The listing builds one solid part. Answer for the finished solid, in the listing's coordinates (mm). Coordinates: 2 decimals unless noted, no trailing zeros. Loops run counter-clockwise (first coordinate to the right, second up) from the corner with the lowest first, then second, coordinate; pieces in that order, holes last. Notation, with made-up numbers: M 3,36.5 L 9,36.5 A17 ccw 9,51.5 Z; hole C 4.5,-18.5 d7. An arc over 180 degrees is marked long. Answer as a JSON object with one key per item and string values. Group by question number.
1. A cutting plane is placed at C-C on x = -40.5. Give the vertices of the cut face in (y, z).
2. Straight lines are drawn through the part: L1, parallel to Z at x = -2, y = 1.25; L2, parallel to Y at x = 7, z = -9; L3, parallel to Z at x = -8, y = 8.75. For each, find the intervals that lie inside material, in ascending order.
3. A cutting plane is placed at A-A on z = 0. Give the vertices of the cut face in (x, y).
4. A cutting plane is placed at B-B on y = 10. Give the vertices of the cut face in (x, z), and give its area (3 significant figures).
5. Given pin 1 (5 mm diameter, centred on x = 24, y = 1.5, fed in from -Z); pin 2 (6 mm diameter, centred on x = -27.5, y = 11, fed in from -Z); pin 3 (6 mm diameter, centred on x = 54.5, y = 7, fed in from -Z), each flat-ended and moving along its own axis, determine where each tip first touches the part or whether it passes through.
6. A cutting plane is placed at D-D on x = 33. Give the vertices of the cut face in (y, z), and give its area (3 significant figures).
from build123d import *

# Parameters (mm, degrees)
SKETCH1_R           = 70
BOSS_EXTRUDE1_DEPTH = 13
SKETCH2_R           = 10
CUT_EXTRUDE1_DEPTH  = 100.844879688
SKETCH3_R           = 8.334076576
CUT_EXTRUDE2_DEPTH  = 10.220805
CIRPATTERN1_START   = 2.779195168
CIRPATTERN1_DEPTH   = 10.220804832


# Read off the part's stored shape, not the designer's step: CirPattern1
with BuildPart() as part:
    # Sketch1 → Boss-Extrude1 (new body)
    with BuildSketch(Plane(origin=(0, 0, 0), x_dir=(1, 0, 0), z_dir=(0, 1, 0))):
        with Locations(Location((0, 0, 0), (0, 0, 90))):
            Circle(SKETCH1_R)
    extrude(amount=BOSS_EXTRUDE1_DEPTH)

    # Sketch2 → Cut-Extrude1 (cut, through all)
    with BuildSketch(Plane(origin=(0, 0, 0), x_dir=(1, 0, 0), z_dir=(0, 1, 0))):
        with Locations(Location((0, 0, 0), (0, 0, 90))):
            Circle(SKETCH2_R)
    extrude(amount=CUT_EXTRUDE1_DEPTH, mode=Mode.SUBTRACT)

    # Sketch3 → Cut-Extrude2 (cut)
    with BuildSketch(Plane(origin=(0, 13, 0), x_dir=(1, 0, 0), z_dir=(0, 1, 0))):
        with Locations((-16.463436294, 0)):
            Circle(SKETCH3_R)
    extrude(amount=-CUT_EXTRUDE2_DEPTH, mode=Mode.SUBTRACT)

    # CirPattern1 outline → CirPattern1 (cut)
    with BuildSketch(Plane(origin=(0, 0, 0), x_dir=(1, 0, 0), z_dir=(0, 1, 0)).offset(CIRPATTERN1_START)):
        with BuildLine():
            ThreePointArc((8.05530373, -5.925544854), (5, -8.660254038), (1.104020509, -9.938870092))
            ThreePointArc((1.104020509, -9.938870092), (0.405285183, -11.39353001), (0, -12.955583291))
            ThreePointArc((0, -12.955583291), (-0.405285183, -11.39353001), (-1.104020509, -9.938870092))
            ThreePointArc((-1.104020509, -9.938870092), (-5, -8.660254038), (-8.05530373, -5.925544854))
            ThreePointArc((-8.05530373, -5.925544854), (-9.664443836, -6.047752269), (-11.219864251, -6.477791645))
            ThreePointArc((-11.219864251, -6.477791645), (-12.296398006, -7.217522031), (-13.475290189, -7.779962418))
            ThreePointArc((-13.475290189, -7.779962418), (-12.398756435, -21.475276095), (0, -15.559924837))
            ThreePointArc((0, -15.559924837), (12.398756435, -21.475276095), (13.475290189, -7.779962418))
            ThreePointArc((13.475290189, -7.779962418), (24.797512869, 0), (13.475290189, 7.779962418))
            ThreePointArc((13.475290189, 7.779962418), (12.398756435, 21.475276095), (0, 15.559924837))
            ThreePointArc((0, 15.559924837), (-12.398756435, 21.475276095), (-13.475290189, 7.779962418))
            ThreePointArc((-13.475290189, 7.779962418), (-12.296398006, 7.217522031), (-11.219864251, 6.477791645))
            ThreePointArc((-11.219864251, 6.477791645), (-9.664443836, 6.047752269), (-8.05530373, 5.925544854))
            ThreePointArc((-8.05530373, 5.925544854), (-5, 8.660254038), (-1.104020509, 9.938870092))
            ThreePointArc((-1.104020509, 9.938870092), (-0.405285183, 11.39353001), (0, 12.955583291))
            ThreePointArc((0, 12.955583291), (0.405285183, 11.39353001), (1.104020509, 9.938870092))
            ThreePointArc((1.104020509, 9.938870092), (5, 8.660254038), (8.05530373, 5.925544854))
            ThreePointArc((8.05530373, 5.925544854), (9.664443836, 6.047752269), (11.219864251, 6.477791645))
            ThreePointArc((11.219864251, 6.477791645), (10.069729019, 5.345777741), (9.15932424, 4.013325239))
            ThreePointArc((9.15932424, 4.013325239), (10, 0), (9.15932424, -4.013325239))
            ThreePointArc((9.15932424, -4.013325239), (10.069729019, -5.345777741), (11.219864251, -6.477791645))
            ThreePointArc((11.219864251, -6.477791645), (9.664443836, -6.047752269), (8.05530373, -5.925544854))
        make_face()
    extrude(amount=CIRPATTERN1_DEPTH, mode=Mode.SUBTRACT)


solid = part.part
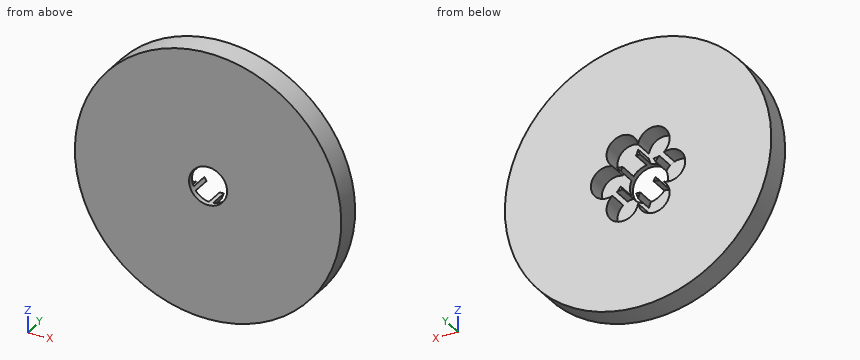
From the geometry:
{
 "1": {"outline": "M 0,-57.09 L 13,-57.09 L 13,57.09 L 0,57.09 Z"},
 "2": {"L1": "z = -69.97 to -9.8, 9.8 to 69.97", "L2": "y = 0 to 2.78", "L3": "z = -69.54 to -22.59, 22.59 to 69.54"},
 "3": {"outline": "M -70,0 L -10,0 L -10,2.78 L -24.8,2.78 L -24.8,13 L -70,13 Z; M 10,0 L 70,0 L 70,13 L 24.8,13 L 24.8,2.78 L 10,2.78 Z"},
 "4": {"outline": "C 0,0 d140; M -11.22,-6.48 A8.33 cw -8.06,-5.93 A10 cw -9.16,-4.01 A8.33 cw Z; M -11.22,6.48 A8.33 cw -9.16,4.01 A10 cw -8.06,5.93 A8.33 cw Z; M -1.1,-9.94 A8.33 cw 0,-12.96 A8.33 cw 1.1,-9.94 A10 cw Z; M -1.1,9.94 A10 cw 1.1,9.94 A8.33 cw 0,12.96 A8.33 cw Z; M 8.06,-5.93 A8.33 cw 11.22,-6.48 A8.33 cw 9.16,-4.01 A10 cw Z; M 8.06,5.93 A10 cw 9.16,4.01 A8.33 cw 11.22,6.48 A8.33 cw Z; hole M -13.48,-7.78 A8.33 ccw long 0,-15.56 A8.33 ccw long 13.48,-7.78 A8.33 ccw long 13.48,7.78 A8.33 ccw long 0,15.56 A8.33 ccw long -13.48,7.78 A8.33 ccw long Z", "area": "13,800 mm²"},
 "5": {"pin 1": "stops at z = -66.62", "pin 2": "stops at z = -65.57", "pin 3": "stops at z = -47.41"},
 "6": {"outline": "M 0,-61.73 L 13,-61.73 L 13,61.73 L 0,61.73 Z", "area": "1,610 mm²"}
}
